Here's how the part is built. I have some questions about the finished solid (model axes, mm). A direction names the side the tool comes from. Round coordinates to 2 decimals unless told otherwise and drop trailing zeros. Loops run counter-clockwise (first coordinate to the right, second up) from the corner with the lowest first, then second, coordinate; pieces in that order, holes last. Notation, with made-up numbers: M -25,-31 L 29,-31 A19 ccw 29,-6 Z; hole C 16,59 d5. An arc over 180 degrees is marked long. Answer as a JSON object with one key per item and string values.
from build123d import *

# Parameters (mm, degrees)
SKETCH1_W                                     = 30
SKETCH1_H                                     = 120
BOSS_EXTRUDE1_DEPTH                           = 9
BOSS_EXTRUDE2_DEPTH                           = 1
CBORE_FOR_M6_HEX_SOCKET_HEAD_CAP1_D           = 6.6
CBORE_FOR_M6_HEX_SOCKET_HEAD_CAP1_CBORE_D     = 11
CBORE_FOR_M6_HEX_SOCKET_HEAD_CAP1_CBORE_DEPTH = 6
SKETCH17_W                                    = 6
SKETCH17_H                                    = 2
BOSS_EXTRUDE3_DEPTH                           = 1
CUT_EXTRUDE11_DEPTH                           = 120.609404064
CUT_EXTRUDE11_DEPTH_BACK                      = 120.609404064
SKETCH18_W                                    = 16
SKETCH18_H                                    = 10
SKETCH19_W                                    = 30
SKETCH19_H                                    = 73
CUT_EXTRUDE12_DEPTH                           = 6
SKETCH20_W                                    = 2
SKETCH20_H                                    = 5
REVOLVE2_ANGLE                                = 90


with BuildPart() as part:
    # Sketch1 → Boss-Extrude1 (new body)
    with BuildSketch(Plane(origin=(0, 0, 0), x_dir=(1, 0, 0), z_dir=(0, 1, 0))):
        with Locations((2.137715261, -58.032657583)):
            Rectangle(SKETCH1_W, SKETCH1_H)
    extrude(amount=BOSS_EXTRUDE1_DEPTH)

    # Sketch2 → Boss-Extrude2 (add)
    with BuildSketch(Plane(origin=(0, 9, 0), x_dir=(1, 0, 0), z_dir=(0, 1, 0))):
        Polygon((-12.862284739, -118.032657583), (17.137715261, -118.032657583), (17.137715261, -68.032657583), (17.137715261, 1.967342417), (12.137715261, 1.967342417), (12.137715261, -113.032657583), (-7.862284739, -113.032657583), (-7.862284739, 1.967342417), (-12.862284739, 1.967342417), (-12.862284739, -73.032657583), align=None)
    extrude(amount=BOSS_EXTRUDE2_DEPTH)

    # CBORE for M6 Hex Socket Head Cap1 (through all)
    with Locations(Plane(origin=(0, 9, 0), x_dir=(1, 0, 0), z_dir=(0, 1, 0))):
        with Locations((2.137715261, -8.032657583), (2.137715261, -33.032657583)):
            CounterBoreHole(CBORE_FOR_M6_HEX_SOCKET_HEAD_CAP1_D / 2, CBORE_FOR_M6_HEX_SOCKET_HEAD_CAP1_CBORE_D / 2, CBORE_FOR_M6_HEX_SOCKET_HEAD_CAP1_CBORE_DEPTH)

    # Sketch17 → Boss-Extrude3 (add)
    with BuildSketch(Plane(origin=(0, 10, 0), x_dir=(1, 0, 0), z_dir=(0, 1, 0))):
        with Locations((14.137715261, -110.032657583)):
            Rectangle(SKETCH17_W, SKETCH17_H)
        with Locations((-9.862284739, -110.032657583)):
            Rectangle(SKETCH17_W, SKETCH17_H)
        with Locations((14.137715261, -103.032657583)):
            Rectangle(SKETCH17_W, SKETCH17_H)
        with Locations((-9.862284739, -103.032657583)):
            Rectangle(SKETCH17_W, SKETCH17_H)
    extrude(amount=BOSS_EXTRUDE3_DEPTH)

    # Sketch18 → Cut-Extrude11 (cut, two sides: drawn at the far end of the back side and taken through both)
    with BuildSketch(Plane(origin=(0, 9, 0), x_dir=(1, 0, 0), z_dir=(0, 1, 0)).offset(-CUT_EXTRUDE11_DEPTH_BACK)):
        with Locations((2.137715261, -106.032657583)):
            Rectangle(SKETCH18_W, SKETCH18_H)
    extrude(amount=CUT_EXTRUDE11_DEPTH + CUT_EXTRUDE11_DEPTH_BACK, mode=Mode.SUBTRACT)

    # Sketch19 → Cut-Extrude12 (cut)
    with BuildSketch(Plane.XZ):
        with Locations((2.137715261, 81.532657583)):
            Rectangle(SKETCH19_W, SKETCH19_H)
    extrude(amount=-CUT_EXTRUDE12_DEPTH, mode=Mode.SUBTRACT)

    # Sketch20 → Revolve2 (revolve)
    with BuildSketch(Plane.XZ.offset(-6)):
        with Locations((-9.862284739, 47.532657583)):
            Rectangle(SKETCH20_W, SKETCH20_H)
        with Locations((14.137715261, 47.532657583)):
            Rectangle(SKETCH20_W, SKETCH20_H)
    revolve(axis=Axis((17.137715261, 6, 45.032657583), (1, 0, 0)), revolution_arc=REVOLVE2_ANGLE)


solid = part.part
Item 1: If I drill on L1, parallel to Z at x = 8.75, y = 7.75; L2, parallel to Z at x = -1, y = 7; L3, parallel to Z at x = -0.25, y = 8.5, over which ranges is the centre line in solid material (lowest first)? Write a range as from..to.
Solution:
{"L1": "z = -1.97..101.03, 111.03..118.03", "L2": "z = -1.97..3.52, 12.55..28.52, 37.55..101.03, 111.03..118.03", "L3": "z = -1.97..3.08, 12.99..28.08, 37.99..101.03, 111.03..118.03"}
Item 2: For P1, Ø9, axis at x = -2, z = 67.5, coming from the -Y side; P2, Ø1.5, axis at y = 3.5, z = 48.5, coming from the +X side; P3, Ø0.8, axis at x = -9.5, y = 10.5, coming from the +Z side, each with a flat end and sliding along its axis, tell me the tip position at first contact or that it passes through.
Solution:
{"P1": "stops at y = 6", "P2": "stops at x = 15.14", "P3": "stops at z = 111.03"}
Item 3: I want a section at D-D on z = 97.5. List the corners of the cut face in (x, y) for me.
Solution:
{"outline": "M -12.86,6 L 17.14,6 L 17.14,10 L 12.14,10 L 12.14,9 L -7.86,9 L -7.86,10 L -12.86,10 Z"}
Item 4: For faces 1 (the face through (2, 3, 45.033)), 2 (the face through (10.138, 7, 106)), 3 (the face through (15, 10, 106)), which set-ups out of +Z, -Z, +X, -X, +Y, -Y let a thin tool reach every point of the face, with its end or its side?
Solution:
{"face 1": "+Z, -Y", "face 2": "+Y, -Y", "face 3": "+X, -X, +Y"}
Item 5: I want a section at B-B on z = 17. List the corners of the cut face in (x, y) for me.
Solution:
{"outline": "M -12.86,0 L 17.14,0 L 17.14,10 L 12.14,10 L 12.14,9 L -7.86,9 L -7.86,10 L -12.86,10 Z"}
Item 6: I want a section at A-A on x = 1.25. List the corners of the cut face in (y, z) for me.
Solution:
{"outline": "M 0,-1.97 L 9,-1.97 L 9,2.6 L 3,2.6 L 3,4.85 L 0,4.85 Z; M 0,11.21 L 3,11.21 L 3,13.46 L 9,13.46 L 9,27.6 L 3,27.6 L 3,29.85 L 0,29.85 Z; M 0,36.21 L 3,36.21 L 3,38.46 L 9,38.46 L 9,101.03 L 6,101.03 L 6,45.03 L 0,45.03 Z; M 6,111.03 L 9,111.03 L 9,113.03 L 10,113.03 L 10,118.03 L 6,118.03 Z"}
Item 7: We'd pull the mould along X, two halves only. Please class faces 4 (the face through (2, 0, 21)), 5 (the face through (-10.862, 4, 47)), 6 (the face through (0.945, 6.042, 13.402)): +X half, -X half, draft (parallel to the pull), parting line (faces both ways), or undercut.
Solution:
{"face 4": "draft", "face 5": "-X half", "face 6": "undercut"}
Item 8: I want a section at C-C on y = 4.25. List the corners of the cut face in (x, z) for me.
Solution:
{"outline": "M -12.86,-1.97 L 17.14,-1.97 L 17.14,45.03 L 15.14,45.03 L 15.14,49.72 L 13.14,49.72 L 13.14,45.03 L -8.86,45.03 L -8.86,49.72 L -10.86,49.72 L -10.86,45.03 L -12.86,45.03 Z; hole C 2.14,8.03 d11; hole C 2.14,33.03 d11"}
